For this review, take the finished solid that the model builds, in its own axes (mm). Round coordinates to 2 decimals unless told otherwise and drop trailing zeros. Order: outer loops, then holes, each group sorted by start corner. A loop starts at its lowest first (then second) coordinate and runs counter-clockwise, first axis right, second up. Notation, with made-up numbers: M -4,3.5 L 18,3.5 A16 cw 18,20.5 Z; hole C 43,72 d7. An arc over 180 degrees is marked long. Use a Markdown table: item, result.
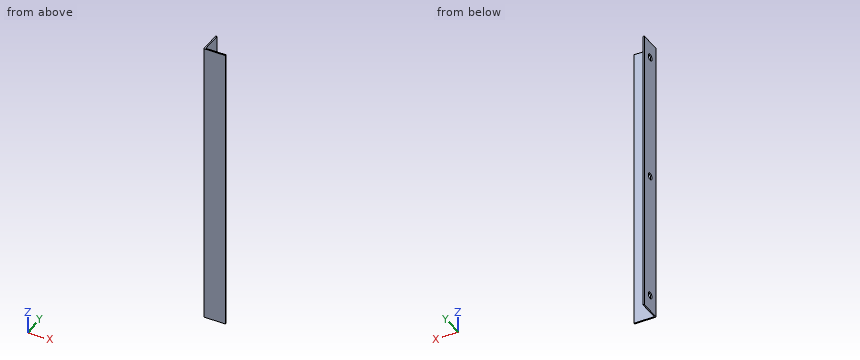
from build123d import *

# Parameters (mm, degrees)
SALIENTE_EXTRUIR1_DEPTH = 338.4
CROQUIS2_R              = 4
CORTAR_EXTRUIR1_DEPTH   = 2


with BuildPart() as part:
    # Croquis1 → Saliente-Extruir1 (new body)
    with BuildSketch(Plane.XY):
        Polygon((0, 0), (0, 25.4), (1.5, 25.4), (1.5, 1.5), (25.4, 1.5), (25.4, 0), align=None)
    extrude(amount=SALIENTE_EXTRUIR1_DEPTH)

    # Croquis2 → Cortar-Extruir1 (cut)
    with BuildSketch(Plane(origin=(1.5, 0, 0), x_dir=(0, 0, -1), z_dir=(1, 0, 0))):
        with Locations((-19.2, 12.9)):
            Circle(CROQUIS2_R)
        with Locations((-319.2, 12.9)):
            Circle(CROQUIS2_R)
        with Locations((-169.2, 12.9)):
            Circle(CROQUIS2_R)
    extrude(amount=-CORTAR_EXTRUIR1_DEPTH, mode=Mode.SUBTRACT)


solid = part.part
Q1. Add section A-A (z = 319.2). Write out the cut boundary in (x, y).
Determined:
| item | result |
|---|---|
| outline | M 0,0 L 25.4,0 L 25.4,1.5 L 1.5,1.5 L 1.5,8.9 L 0,8.9 Z; M 0,16.9 L 1.5,16.9 L 1.5,25.4 L 0,25.4 Z |
Q2. Add section B-B (y = 12.9). Write out the cut boundary in (x, z), then the cut area to 3 significant figures.
Determined:
| item | result |
|---|---|
| outline | M 0,0 L 1.5,0 L 1.5,15.2 L 0,15.2 Z; M 0,23.2 L 1.5,23.2 L 1.5,165.2 L 0,165.2 Z; M 0,173.2 L 1.5,173.2 L 1.5,315.2 L 0,315.2 Z; M 0,323.2 L 1.5,323.2 L 1.5,338.4 L 0,338.4 Z |
| area | 472 mm^2 |
Q3. Wall thickness on line 1 along Y through (x, z) = (1.2, 169.2); line 2 along Y through (x, z) = (23, 308): over which ranges is each line inside the solid? List them lowest first. Write a range as [from, to].
Determined:
| item | result |
|---|---|
| line 1 | y = [0, 8.9], [16.9, 25.4] |
| line 2 | y = [0, 1.5] |
Q4. Clearance check with flat-ended pins moving along their axes: pin 1 (10.5 mm diameter, centred on y = 12.9, z = 19.2, fed in from +X); pin 2 (3 mm diameter, centred on x = 18, z = 112, fed in from +Y); pin 3 (5 mm diameter, centred on y = 12.9, z = 169.2, fed in from +X). State where each tip first meets the part, or that it passes through.
Determined:
| item | result |
|---|---|
| pin 1 | stops at x = 1.5 |
| pin 2 | stops at y = 1.5 |
| pin 3 | passes through |
Q5. Add section D-D (x = 16.25). Write out the cut boundary in (y, z).
Determined:
| item | result |
|---|---|
| outline | M 0,0 L 1.5,0 L 1.5,338.4 L 0,338.4 Z |
Q6. Add section C-C (z = 194). Write out the cut boundary in (x, y).
Determined:
| item | result |
|---|---|
| outline | M 0,0 L 25.4,0 L 25.4,1.5 L 1.5,1.5 L 1.5,25.4 L 0,25.4 Z |
